from build123d import *

# Parameters (mm, degrees)
SKETCH1_W           = 76.2
SKETCH1_H           = 57.15
SKETCH1_R           = 6.35
BOSS_EXTRUDE1_DEPTH = 101.6
SKETCH2_W           = 50.8
SKETCH2_H           = 25.4
CUT_EXTRUDE1_DEPTH  = 19.05
SKETCH3_W           = 25.4
SKETCH3_H           = 50.8
CUT_EXTRUDE2_DEPTH  = 19.05
SKETCH4_R           = 6.35
BOSS_EXTRUDE2_DEPTH = 2.54
FILLET1_R           = 31.75


with BuildPart() as part:
    # Sketch1 → Boss-Extrude1 (new body)
    with BuildSketch(Plane.XY):
        with Locations((-4.930961298, 9.873813983)):
            Rectangle(SKETCH1_W, SKETCH1_H)
        with Locations((7.769038702, 0.348813983)):
            Circle(SKETCH1_R, mode=Mode.SUBTRACT)
    extrude(amount=BOSS_EXTRUDE1_DEPTH)

    # Sketch2 → Cut-Extrude1 (cut)
    with BuildSketch(Plane.ZY.offset(43.030961298)):
        with Locations((31.75, 9.873813983)):
            Rectangle(SKETCH2_W, SKETCH2_H)
    extrude(amount=-CUT_EXTRUDE1_DEPTH, mode=Mode.SUBTRACT)

    # Sketch3 → Cut-Extrude2 (cut)
    with BuildSketch(Plane.XY.offset(101.6)):
        with Locations((-23.980961298, 9.873813983)):
            Rectangle(SKETCH3_W, SKETCH3_H)
    extrude(amount=-CUT_EXTRUDE2_DEPTH, mode=Mode.SUBTRACT)

    # Sketch4 → Boss-Extrude2 (add)
    with BuildSketch(Plane.ZY.offset(23.980961298)):
        with Locations(Location((44.45, 9.873813983, 0), (0, 0, 270))):
            Circle(SKETCH4_R)
    extrude(amount=BOSS_EXTRUDE2_DEPTH)

    # Fillet1
    fillet1_edges = [part.edges().sort_by_distance(p)[0] for p in [
        (33.169038702, 38.448813983, 50.8),
    ]]
    fillet(fillet1_edges, radius=FILLET1_R)


solid = part.part
Could you check a few things on this model? Use its own coordinates, in mm. A direction names the side the tool comes from. Give positions to 0.01 mm unless a question says otherwise; leave off trailing zeros. Order: outer loops, then holes, each group sorted by start corner. A loop starts at its lowest first (then second) coordinate and runs counter-clockwise, first axis right, second up.
1. I need wall thicknesses on L1, parallel to Y at x = -37.5, z = 19.5; L2, parallel to Z at x = -26, y = 12; L3, parallel to Z at x = -30, y = 33. Which ranges of each line are inside material? Lowest first, please.
2. Suppose I cut it at B-B (z = 44.45). List the corners of the cut face in (x, y) for me.
3. Suppose I cut it at A-A (x = -35). List the corners of the cut face in (y, z) for me, plus the area to 3 significant figures.
4. Will these pins go through, and if not, where does the flat tip stop? P1, Ø6.5, axis at y = 7, z = 44.5, coming from the -X side; P2, Ø2, axis at y = 11.5, z = 46, coming from the +X side; P3, Ø1.5, axis at x = 20, z = 90.5, coming from the +Y side.
5. For faces 1 (the flat face through (-23.981, 10, 31)), 2 (the flat face through (33.169, -6, 50)), 3 (the flat face through (-11.281, 10, 92)), which set-ups out of +Z, -Z, +X, -X, +Y, -Y let a thin tool reach every point of the face, with its end or its side?
6. Suppose I cut it at D-D (y = 14). List the corners of the cut face in (x, z) for me.
7. We'd pull the mould along Y, two halves only. Please class faces 4 (the cylindrical face through (23.621, 29.395, 51.511)), 5 (the flat face through (-34, 10, 6.35)), 6 (the flat face through (-43.031, 9, 61)): pulls with the +Y half, pulls with the -Y half, needs draft (parallel to the pull), parting line crosses it, or undercut.
8. Suppose I cut it at C-C (y = 5). List the corners of the cut face in (x, z) for me.
Solved:
1. L1: y = -18.7 to -2.83, 22.57 to 38.45
1. L2: z = 0 to 6.35, 38.47 to 50.43, 57.15 to 82.55
1. L3: z = 0 to 82.55
2. outline: (-43.03, -18.7) - (33.17, -18.7) - (33.17, 6.7) arc R31.75 ccw to (1.42, 38.45) - (-43.03, 38.45) - (-43.03, 22.57) - (-23.98, 22.57) - (-23.98, 16.22) - (-26.52, 16.22) - (-26.52, 3.52) - (-23.98, 3.52) - (-23.98, -2.83) - (-43.03, -2.83) - close; hole circle Ø12.7 at (7.77, 0.35)
3. outline: (-18.7, 0) - (38.45, 0) - (38.45, 101.6) - (35.27, 101.6) - (35.27, 82.55) - (-15.53, 82.55) - (-15.53, 101.6) - (-18.7, 101.6) - close; hole (-2.83, 6.35) - (22.57, 6.35) - (22.57, 57.15) - (-2.83, 57.15) - close
3. area: 3,550 mm2
4. P1: stops at x = -26.52
4. P2: stops at x = 32.94
4. P3: stops at y = 32.97
5. face 1: -X
5. face 2: +Z, -Z, +X, +Y, -Y
5. face 3: +Z
6. outline: (-43.03, 0) - (32.32, 0) - (32.32, 101.6) - (-11.28, 101.6) - (-11.28, 82.55) - (-36.68, 82.55) - (-36.68, 101.6) - (-43.03, 101.6) - (-43.03, 57.15) - (-23.98, 57.15) - (-23.98, 49.28) - (-26.52, 49.28) - (-26.52, 39.62) - (-23.98, 39.62) - (-23.98, 6.35) - (-43.03, 6.35) - close
7. face 4: pulls with the +Y half
7. face 5: undercut
7. face 6: needs draft
8. outline: (-43.03, 0) - (3.45, 0) - (3.45, 101.6) - (-11.28, 101.6) - (-11.28, 82.55) - (-36.68, 82.55) - (-36.68, 101.6) - (-43.03, 101.6) - (-43.03, 57.15) - (-23.98, 57.15) - (-23.98, 48.52) - (-26.52, 48.52) - (-26.52, 40.38) - (-23.98, 40.38) - (-23.98, 6.35) - (-43.03, 6.35) - close; (12.09, 0) - (33.17, 0) - (33.17, 101.6) - (12.09, 101.6) - close
